from build123d import *

# Parameters (mm, degrees)
SKETCH1_R           = 18.75
SKETCH1_R_2         = 12.5
BOSS_EXTRUDE1_DEPTH = 10
SKETCH1_3_R         = 18.75
SKETCH1_3_R_2       = 12.5
BOSS_EXTRUDE2_DEPTH = 5


with BuildPart() as part:
    # Sketch1 → Boss-Extrude1 (new, symmetric)
    with BuildSketch(Plane(origin=(0, 0, 0), x_dir=(1, 0, 0), z_dir=(0, 1, 0))):
        with BuildLine():
            Line((-71.875, -37.369564822), (77.083333333, -24.913043215))
            ThreePointArc((77.083333333, -24.913043215), (100, 0), (77.083333333, 24.913043215))
            Line((77.083333333, 24.913043215), (-71.875, 37.369564822))
            ThreePointArc((-71.875, 37.369564822), (-112.5, 0), (-71.875, -37.369564822))
        make_face()
        with Locations(Location((75, 0, 0), (0, 0, 270))):
            Circle(SKETCH1_R, mode=Mode.SUBTRACT)
        with Locations(Location((-75, 0, 0), (0, 0, 270))):
            Circle(SKETCH1_R_2, mode=Mode.SUBTRACT)
    extrude(amount=BOSS_EXTRUDE1_DEPTH, both=True)

    # Sketch1_3 → Boss-Extrude2 (add, symmetric)
    with BuildSketch(Plane(origin=(0, 0, 0), x_dir=(1, 0, 0), z_dir=(0, 1, 0))):
        with Locations(Location((75, 0, 0), (0, 0, 270))):
            Circle(SKETCH1_3_R)
        with Locations(Location((75, 0, 0), (0, 0, 270))):
            Circle(SKETCH1_3_R_2, mode=Mode.SUBTRACT)
    extrude(amount=BOSS_EXTRUDE2_DEPTH, both=True)


solid = part.part
Design review of the part built by this model. Coordinates are the model's own, in mm. A direction names the side the tool comes from. Give positions to 0.01 mm unless a question says otherwise; leave off trailing zeros. Order: outer loops, then holes, each group sorted by start corner. A loop starts at its lowest first (then second) coordinate and runs counter-clockwise, first axis right, second up.
1. For pin 1 Ø1.5 at (y, z) = (6.5, 5.5) entering from +X; pin 2 Ø19 at (x, z) = (76, -8) entering from +Y; pin 3 Ø15 at (x, z) = (-75, 0) entering from -Y; pin 4 Ø4 at (y, z) = (-6.5, -21.5) entering from +X, all flat-tipped, find the tip position at first contact; note any pin that passes through.
Solution:
pin 1: stops at x = 99.54
pin 2: stops at y = 5
pin 3: passes through
pin 4: stops at x = 90.64
2. Add section A-A, the plane x = -75. State the section outline as (y, z) points, then the cut area to 4 significant figures.
Solution:
outline: (-10, -37.5) - (10, -37.5) - (10, -12.5) - (-10, -12.5) - close; (-10, 12.5) - (10, 12.5) - (10, 37.5) - (-10, 37.5) - close
area: 1,000 mm2
3. Mouldability with a two-part tool opening along Z and no side actions: class faces 1 (the flat face through (71.1, 5, 12.2)), 2 (the flat face through (-31, -10, -1)), 3 (the flat face through (1.56, 0.14, 31.23)) as +Z half, -Z half, draft (parallel to the pull), parting line (faces both ways), or undercut.
Solution:
face 1: undercut
face 2: draft
face 3: +Z half
4. Add section C-C, the plane y = 3. State the section outline as (x, z) points (3 decimals), then the cut area to 3 significant figures.
Solution:
outline: (-71.875, -37.37) - (77.083, -24.913) arc R25 ccw to (77.083, 24.913) - (-71.875, 37.37) arc R37.5 ccw (long way) to start; hole circle Ø25 at (-75, 0); hole circle Ø25 at (75, 0)
area: 11,600 mm2
5. To check wall thickness, follow L1, parallel to X at y = -2.25, z = 8.5; L2, parallel to Z at x = -64, y = 7.25; L3, parallel to Z at x = -32, y = -5.5. State the ranges of each line that lie inside material, in increasing order.
Solution:
L1: x = -111.52 to -84.17, -65.83 to 65.83, 84.17 to 98.51
L2: z = -36.71 to -5.94, 5.94 to 36.71
L3: z = -34.04 to 34.04
6. Add section B-B, the plane z = 0. State the section outline as (x, y) points, then the cut area to 4 significant figures.
Solution:
outline: (-112.5, -10) - (-87.5, -10) - (-87.5, 10) - (-112.5, 10) - close; (-62.5, -10) - (56.25, -10) - (56.25, -5) - (62.5, -5) - (62.5, 5) - (56.25, 5) - (56.25, 10) - (-62.5, 10) - close; (87.5, -5) - (93.75, -5) - (93.75, -10) - (100, -10) - (100, 10) - (93.75, 10) - (93.75, 5) - (87.5, 5) - close
area: 3,125 mm2
7. Add section D-D, the plane x = 75. State the section outline as (y, z) points, then the cut area to 3 significant figures.
Solution:
outline: (-10, -25.09) - (10, -25.09) - (10, -18.75) - (5, -18.75) - (5, -12.5) - (-5, -12.5) - (-5, -18.75) - (-10, -18.75) - close; (-10, 18.75) - (-5, 18.75) - (-5, 12.5) - (5, 12.5) - (5, 18.75) - (10, 18.75) - (10, 25.09) - (-10, 25.09) - close
area: 378 mm2
8. Tool access review of faces 4 (the cylindrical face through (-62.606, -0.14, -1.627)), 5 (the cylindrical face through (93.59, 7.46, -2.44)), 6 (the cylindrical face through (93.59, -7.54, -2.44)): name each direction out of +Z, -Z, +X, -X, +Y, -Y from which nothing blocks a thin tool from reaching the whole face with its end or side.
Solution:
face 4: +Y, -Y
face 5: +Y
face 6: -Y
